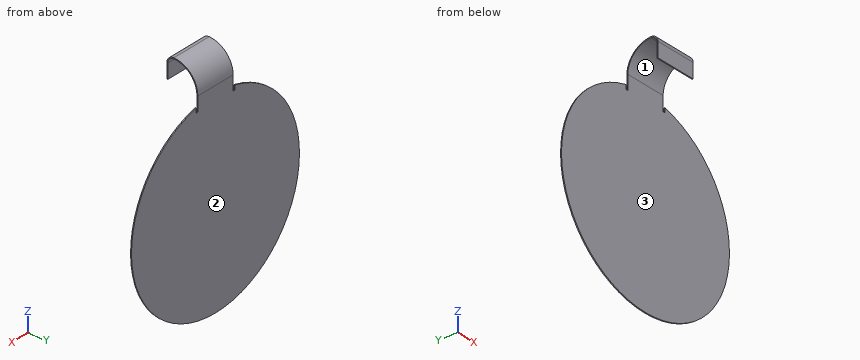
from build123d import *

# Parameters (mm, degrees)
SKETCH1_R                       = 10
BOSS_EXTRUDE1_DEPTH             = 0.1
BOSS_EXTRUDE2_START             = -2
SKETCH3_W                       = 4.2
SKETCH3_H                       = 1
BOSS_EXTRUDE2_DEPTH             = 0.1
EXTRUDE_THIN1_REACH             = 17.393
EXTRUDE_THIN1_DIRECTION_2_REACH = 17.393
SKETCH5_W                       = 0.2
SKETCH5_H                       = 0.5
CUT_EXTRUDE1_DEPTH              = 0.1


with BuildPart() as part:
    # Sketch1 → Boss-Extrude1 (new body)
    with BuildSketch(Plane(origin=(0, 1.1, 0), x_dir=(1, 0, 0), z_dir=(0, 1, 0))):
        with Locations(Location((0, 1.53064501, 0), (0, 0, 270))):
            Circle(SKETCH1_R)
    extrude(amount=BOSS_EXTRUDE1_DEPTH)


with BuildPart() as body_2:
    # Sketch3 → Boss-Extrude2 (new body)
    with BuildSketch(Plane(origin=(0, 0, 0), x_dir=(1, 0, 0), z_dir=(0, 1, 0)).offset(BOSS_EXTRUDE2_START)):
        with Locations((0, -10)):
            Rectangle(SKETCH3_W, SKETCH3_H)
    extrude(amount=BOSS_EXTRUDE2_DEPTH)

    # Extrude-Thin1: up to this face of the body (flat: up to its plane)
    extrude_thin1_end = Plane(body_2.part.faces().sort_by_distance((2.1, -1.95, 10))[0])
    # Sketch4 → Extrude-Thin1 (add, up to the picked face)
    with BuildSketch(Plane(origin=(0, 0, 0), x_dir=(0, 0, -1), z_dir=(1, 0, 0)), mode=Mode.PRIVATE) as extrude_thin1_sk1:
        with BuildLine():
            Line((-9.5, -2), (-10.5, -2))
            Line((-10.5, -2), (-11, -2))
            ThreePointArc((-11, -2), (-11.511328882, -1.786579748), (-11.7192089, -1.27297355))
            ThreePointArc((-11.7192089, -1.27297355), (-10.977540685, 0.47729656), (-9.21935499, 1.2))
            Line((-9.21935499, 1.2), (-8.46935499, 1.2))
            Line((-8.46935499, 1.2), (-5, 1.2))
            Line((-5, 1.2), (-5, 1.1))
            Line((-5, 1.1), (-8.46935499, 1.1))
            Line((-8.46935499, 1.1), (-9.21935499, 1.1))
            ThreePointArc((-9.21935499, 1.1), (-10.907213257, 0.406204698), (-11.619214744, -1.274054608))
            ThreePointArc((-11.619214744, -1.274054608), (-11.440237019, -1.716252321), (-11, -1.9))
            Line((-11, -1.9), (-10.5, -1.9))
            Line((-10.5, -1.9), (-9.5, -1.9))
            Line((-9.5, -1.9), (-9.5, -2))
        make_face()
    extrude_thin1_tool1 = split(extrude(extrude_thin1_sk1.sketch, amount=EXTRUDE_THIN1_REACH, mode=Mode.PRIVATE), bisect_by=extrude_thin1_end, keep=Keep.BOTH, mode=Mode.PRIVATE)

    add(part.part)  # Extrude-Thin1 merges part
    add(extrude_thin1_tool1.solids().sort_by(Axis((0, -1.974423, 10.75), (1, 0, 0)))[0])

    # Extrude-Thin1 direction 2: up to this face of the body (flat: up to its plane)
    extrude_thin1_direction_2_end = Plane(body_2.part.faces().sort_by_distance((-2.1, -1.95, 10))[0])
    # Sketch4 → Extrude-Thin1 direction 2 (add, up to the picked face)
    with BuildSketch(Plane(origin=(0, 0, 0), x_dir=(0, 0, -1), z_dir=(1, 0, 0)), mode=Mode.PRIVATE) as extrude_thin1_direction_2_sk1:
        with BuildLine():
            Line((-9.5, -2), (-10.5, -2))
            Line((-10.5, -2), (-11, -2))
            ThreePointArc((-11, -2), (-11.511328882, -1.786579748), (-11.7192089, -1.27297355))
            ThreePointArc((-11.7192089, -1.27297355), (-10.977540685, 0.47729656), (-9.21935499, 1.2))
            Line((-9.21935499, 1.2), (-8.46935499, 1.2))
            Line((-8.46935499, 1.2), (-5, 1.2))
            Line((-5, 1.2), (-5, 1.1))
            Line((-5, 1.1), (-8.46935499, 1.1))
            Line((-8.46935499, 1.1), (-9.21935499, 1.1))
            ThreePointArc((-9.21935499, 1.1), (-10.907213257, 0.406204698), (-11.619214744, -1.274054608))
            ThreePointArc((-11.619214744, -1.274054608), (-11.440237019, -1.716252321), (-11, -1.9))
            Line((-11, -1.9), (-10.5, -1.9))
            Line((-10.5, -1.9), (-9.5, -1.9))
            Line((-9.5, -1.9), (-9.5, -2))
        make_face()
    extrude_thin1_direction_2_tool1 = split(extrude(extrude_thin1_direction_2_sk1.sketch, amount=-EXTRUDE_THIN1_DIRECTION_2_REACH, mode=Mode.PRIVATE), bisect_by=extrude_thin1_direction_2_end, keep=Keep.BOTH, mode=Mode.PRIVATE)
    add(extrude_thin1_direction_2_tool1.solids().sort_by(Axis((0, -1.974423, 10.75), (-1, 0, 0)))[0])

    # Sketch5 → Cut-Extrude1 (cut)
    with BuildSketch(Plane(origin=(0, 1.2, 0), x_dir=(1, 0, 0), z_dir=(0, 1, 0))):
        with Locations((-2.2, -7.996368849)):
            Rectangle(SKETCH5_W, SKETCH5_H)
        with Locations((2.2, -7.996368849)):
            Rectangle(SKETCH5_W, SKETCH5_H)
    extrude(amount=-CUT_EXTRUDE1_DEPTH, mode=Mode.SUBTRACT)


solid = body_2.part
Geometry: final body of the model. Coordinates: model frame, mm. Face numbers are marked on the shaded views. Give positions to 0.01 mm unless a question says otherwise; leave off trailing zeros. Order: outer loops, then holes, each group sorted by start corner. A loop starts at its lowest first (then second) coordinate and runs counter-clockwise, first axis right, second up. Notation, with made-up numbers: (-18.75, -19.5) -> (37.25, -19.5) arc R15 ccw to (37.25, -8.5) -> close; hole circle Ø5 at (62, -4.5). An arc over 180 degrees is marked (long way). Answer as a JSON object with one key per item and string values.
Q1. Section C-C (y = -0.25). Output: boundary loops of the cut face in (x, z).
Entries:
{"outline": "(-2.1, 11.38) -> (2.1, 11.38) -> (2.1, 11.49) -> (-2.1, 11.49) -> close"}
Q2. Section A-A (x = 0). Output: boundary loops of the cut face in (y, z).
Entries:
{"outline": "(-2, 9.5) -> (-1.9, 9.5) -> (-1.9, 11) arc R0.62 cw to (-1.27, 11.62) arc R2.4 cw to (1.1, 9.22) -> (1.1, -11.53) -> (1.2, -11.53) -> (1.2, 9.22) arc R2.5 ccw to (-1.27, 11.72) arc R0.72 ccw to (-2, 11) -> close"}
Q3. Draft query along Y for the marked faces 1, 2 and 3. Return one class per face: released by +Y, released by -Y, zero draft, split by the parting line, or undercut.
Entries:
{"face 1": "undercut", "face 2": "released by +Y", "face 3": "released by -Y"}
Q4. Section B-B (z = 2.25). Output: boundary loops of the cut face in (x, y), plus the area to 3 significant figures.
Entries:
{"outline": "(-9.26, 1.1) -> (9.26, 1.1) -> (9.26, 1.2) -> (-9.26, 1.2) -> close", "area": "1.85 mm^2"}
